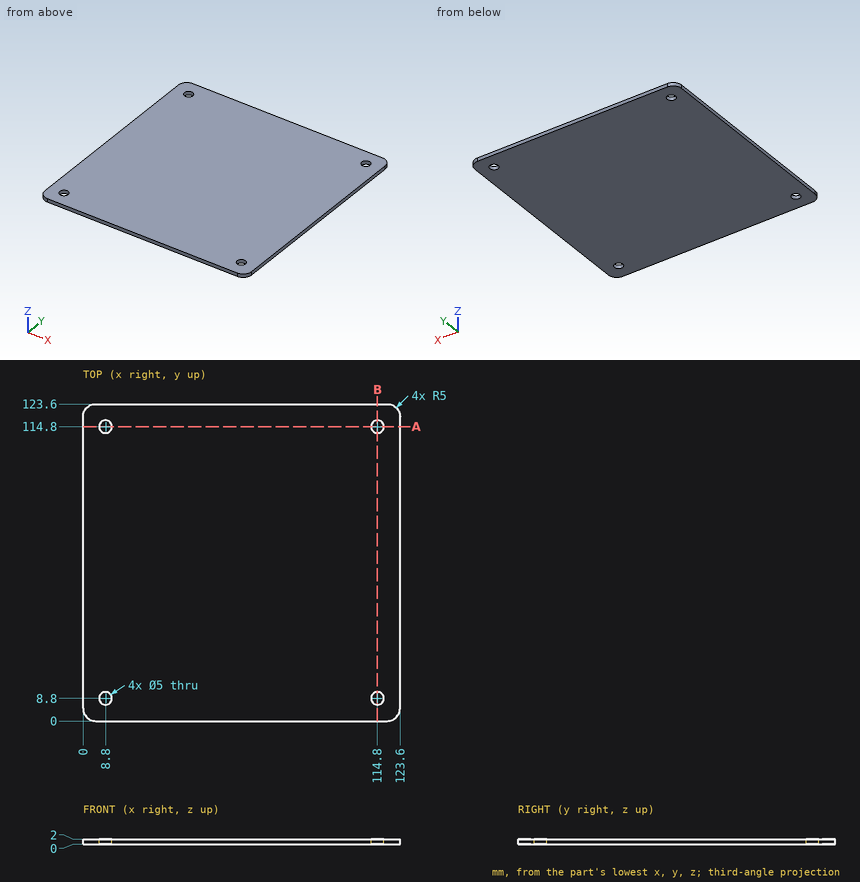
Check sheet for the drawn part. Datum: minimum x, y, z corner. Units: mm. Round coordinates to 2 decimals unless told otherwise and drop trailing zeros. Order: outer loops, then holes, each group sorted by start corner. A loop starts at its lowest first (then second) coordinate and runs counter-clockwise, first axis right, second up. Notation, with made-up numbers: (-24, 3.5) -> (4, 3.5) arc R15 cw to (4, 20.5) -> close; hole circle Ø8 at (61, 17.5). An arc over 180 degrees is marked (long way). Return JSON: item names as keys, results as strings. Group by question number.
Q1. Gauge pin test, flat end, axial feed: pin 1 (6 mm diameter, centred on x = 114.8, y = 8.8, fed in from -Z). Record the tip position at first contact, or that the pin passes through.
Q2. Section check A-A, the plane y = 114.8. Record the boundary of the cut face in (x, z), plus the area to 3 significant figures.
Q3. Material ranges on probe 1 along Y at (x, z) = (8.8, 1.4); probe 2 along X at (y, z) = (114.5, 1.55); probe 3 along X at (y, z) = (113.5, 0.95), recorded low to high. Write a range as from..to.
Numbers:
{
 "1": {"pin 1": "z = 0"},
 "2": {"outline": "(0, 0) -> (6.3, 0) -> (6.3, 2) -> (0, 2) -> close; (11.3, 0) -> (112.3, 0) -> (112.3, 2) -> (11.3, 2) -> close; (117.3, 0) -> (123.6, 0) -> (123.6, 2) -> (117.3, 2) -> close", "area": "227 mm^2"},
 "3": {"probe 1": "0..6.3, 11.3..112.3, 117.3..123.6", "probe 2": "0..6.32, 11.28..112.32, 117.28..123.6", "probe 3": "0..6.66, 10.94..112.66, 116.94..123.6"}
}
